Could you check a few things on this model? Use its own coordinates, in mm. Coordinates: 2 decimals unless noted, no trailing zeros. Write each loop counter-clockwise with the first axis right and the second up, starting at its lowest first coordinate (ties: lowest second). Pieces come first, ordered by that corner, then holes.
Item 1: If I drill on probe 1 along X at (y, z) = (1.5, -17.5); probe 2 along X at (y, z) = (4.25, -16.5); probe 3 along X at (y, z) = (3.5, 25), over which ranges is the centre line in solid material (lowest first)?
Item 2: Thinking about a two-plate mould opening in X: for faces 1 (the cylindrical face through (27.95, 3.91, -0.11)), 2 (the cylindrical face through (-30.995, 3.913, -6.883)), 3 (the flat face through (8, 7.938, -15)), which applies, +X half, -X half, draft (parallel to the pull), parting line (faces both ways), or undercut?
Item 3: I want a section at A-A on z = 25.4. Please give me the cut outline in (x, y).
Item 4: I want a section at C-C on x = -25.4. Please give me the cut outline in (y, z).
Item 5: I want a section at B-B on z = 0. State how many separate pieces and enclosed holes the cut face has, then the cut area to 3 significant figures.
Item 6: For P1, Ø4, axis at x = -17, y = 5.5, coming from the -Z side; P2, Ø1.5, axis at y = 1.5, z = 8, coming from the -X side; P3, Ø1.5, axis at y = 7, z = -1, coming from the +X side, each with a flat end and sliding along its axis, tell me the tip position at first contact or that it passes through.
from build123d import *

# Parameters (mm, degrees)
SKETCH1_R              = 31.75
SKETCH1_R_2            = 15.875
BOSS_EXTRUDE1_DEPTH    = 7.9375
F_10_CLEARANCE_HOLE1_D = 5.1054


with BuildPart() as part:
    # Sketch1 → Boss-Extrude1 (new body)
    with BuildSketch(Plane(origin=(0, 0, 0), x_dir=(1, 0, 0), z_dir=(0, 1, 0))):
        with Locations(Location((0, 0, 0), (0, 0, 270))):
            Circle(SKETCH1_R)
        with Locations(Location((0, 0, 0), (0, 0, 270))):
            Circle(SKETCH1_R_2, mode=Mode.SUBTRACT)
    extrude(amount=BOSS_EXTRUDE1_DEPTH)

    # #10 Clearance Hole1 (through all)
    with Locations(Plane(origin=(0, 7.9375, 0), x_dir=(1, 0, 0), z_dir=(0, 1, 0))):
        with Locations((0, 25.4), (17.960512242, 17.960512242), (25.4, 0), (17.960512242, -17.960512242), (0, -25.4), (-17.960512242, -17.960512242), (-25.4, 0), (-17.960512242, 17.960512242)):
            Hole(F_10_CLEARANCE_HOLE1_D / 2)


solid = part.part
Response values:
1. probe 1: x = -26.49 to -20.47, -15.45 to 15.45, 20.47 to 26.49
1. probe 2: x = -27.13 to -20.05, -15.87 to 15.87, 20.05 to 27.13
1. probe 3: x = -19.57 to -2.52, 2.52 to 19.57
2. face 1: undercut
2. face 2: parting line
2. face 3: draft
3. outline: (-19.05, 0) - (-2.55, 0) - (-2.55, 7.94) - (-19.05, 7.94) - close; (2.55, 0) - (19.05, 0) - (19.05, 7.94) - (2.55, 7.94) - close
4. outline: (0, -19.05) - (7.94, -19.05) - (7.94, -2.55) - (0, -2.55) - close; (0, 2.55) - (7.94, 2.55) - (7.94, 19.05) - (0, 19.05) - close
5. separate pieces: 4
5. enclosed holes: 0
5. area: 171 mm2
6. P1: stops at z = -27.98
6. P2: stops at x = -30.91
6. P3: stops at x = 31.75
